Model file for the job. Use its own axes, mm. A direction names the side the tool comes from. Coordinates: 2 decimals unless noted, no trailing zeros. Order: outer loops, then holes, each group sorted by start corner. A loop starts at its lowest first (then second) coordinate and runs counter-clockwise, first axis right, second up. Notation, with made-up numbers: (-9.75, -4.75) -> (8.25, -4.75) arc R25 ccw to (8.25, 22.25) -> close; hole circle Ø6 at (31, 30). An arc over 180 degrees is marked (long way). Write item = value, one per line. Start each with the question number.
Q1. Flat gauge pins, fed straight in: pin 1 (2 mm diameter, centred on x = -6, z = -8.5, fed in from -Y); pin 2 (7 mm diameter, centred on x = -1.5, y = 2, fed in from -Z); pin 3 (13.5 mm diameter, centred on x = 0, y = 0, fed in from +Z); pin 4 (4 mm diameter, centred on x = 0, y = 0, fed in from -Z). Where does each tip first touch, or does it go through?
Q2. Cut at C-C, the plane z = -10. List the corners of the cut face in (x, y).
Q3. Wall check: line 1 (Y direction, x = 0, z = -17.75); line 2 (Y direction, x = 0, z = 9); line 3 (Z direction, x = 3.5, y = 2.75). Give the ranges that are in metal, low to high. Write a range as from..to.
Q4. 3-axis set-ups, long thin cutter, end or side, ignore diameter. For faces 1 (the face through (-7.493, 0.33, 17.232)), 2 (the face through (1, -3, -16)), 3 (the face through (-8, -2, -19)): which of +Z, -Z, +X, -X, +Y, -Y reach the whole face in a straight line?
Q5. Mould opens along Y. For faces 4 (the face through (-8, -2, 19)), 5 (the face through (-0.54, -2.44, -0.22)), 6 (the face through (11.923, 3.755, 0.252)) say: +Y half, -Y half, draft (parallel to the pull), parting line (faces both ways), or undercut.
from build123d import *

# Parameters (mm, degrees)
SKETCH1_R           = 12.5
SKETCH1_R_2         = 7.5
BOSS_EXTRUDE2_DEPTH = 19
SKETCH1_4_R         = 7.5
SKETCH1_4_R_2       = 2.5
BOSS_EXTRUDE3_DEPTH = 16
CHAMFER1_SIZE       = 1
FILLET1_R           = 0.5
FILLET2_R           = 0.5


with BuildPart() as part:
    # Sketch1 → Boss-Extrude2 (new, symmetric)
    with BuildSketch(Plane.XY):
        Circle(SKETCH1_R)
        Circle(SKETCH1_R_2, mode=Mode.SUBTRACT)
    extrude(amount=BOSS_EXTRUDE2_DEPTH, both=True)

    # Sketch1<4> → Boss-Extrude3 (add, symmetric)
    with BuildSketch(Plane.XY):
        Circle(SKETCH1_4_R)
        Circle(SKETCH1_4_R_2, mode=Mode.SUBTRACT)
    extrude(amount=BOSS_EXTRUDE3_DEPTH, both=True)

    # Chamfer1
    chamfer1_edges = [part.edges().sort_by_distance(p)[0] for p in [
        (-12.5, 0, 19),
        (-12.5, 0, -19),
    ]]
    chamfer(chamfer1_edges, length=CHAMFER1_SIZE)

    # Fillet1
    fillet1_edges = [part.edges().sort_by_distance(p)[0] for p in [
        (-7.5, 0, -16),
        (-2.5, 0, -16),
        (-7.5, 0, -19),
        (-7.5, 0, 19),
    ]]
    fillet(fillet1_edges, radius=FILLET1_R)

    # Fillet2
    fillet2_edges = [part.edges().sort_by_distance(p)[0] for p in [
        (-2.5, 0, 16),
    ]]
    fillet(fillet2_edges, radius=FILLET2_R)


solid = part.part
Here are the results:
q1.pin_1 = -11.46
q1.pin_2 = -16
q1.pin_3 = 16
q1.pin_4 = through
q2.outline = circle Ø25 at (0, 0); hole circle Ø5 at (0, 0)
q3.line_1 = -12.5..-7.5, 7.5..12.5
q3.line_2 = -12.5..-2.5, 2.5..12.5
q3.line_3 = -16..16
q4.face_1 = +Z
q4.face_2 = -Z
q4.face_3 = -Z, +X, -X, +Y, -Y
q5.face_4 = draft
q5.face_5 = undercut
q5.face_6 = parting line
